Part model, mm, in its own coordinate system. Face numbers are marked on the shaded views. Give positions to 0.01 mm unless a question says otherwise; leave off trailing zeros. Order: outer loops, then holes, each group sorted by start corner. A loop starts at its lowest first (then second) coordinate and runs counter-clockwise, first axis right, second up. Notation, with made-up numbers: (-39.5, -39.75) -> (1.5, -39.75) arc R21 cw to (1.5, -32.75) -> close; hole circle Ø1 at (7, 87.5). An arc over 180 degrees is marked (long way). Write item = value, one per line. Start each with the question number.
(1) Two-plate mould, pull along Z, no slides. Class the marked faces 1, 2 and 3: pulls with the +Z half, pulls with the -Z half, needs draft (parallel to the pull), parting line crosses it, or undercut.
(2) Saw through at B-B, the plane x = -10. List the corners of the cut face in (y, z), then the cut area to 3 significant figures.
(3) Saw through at A-A, the plane x = 10. List the corners of the cut face in (y, z), then the cut area to 3 significant figures.
(4) Flat gauge pins, fed straight in: pin 1 (8 mm diameter, centred on x = 10, z = 0, fed in from +Y); pin 2 (3 mm diameter, centred on x = 10.5, z = -14.5, fed in from +Y); pin 3 (12.5 mm diameter, centred on x = 10, z = 0, fed in from -Y). Where does each tip first touch, or does it go through?
(5) Probe line 1 along X through (y, z) = (49, 0); line 2 along X through (y, z) = (47.25, 0); line 3 along Y through (x, z) = (-9.5, -6). List the from-to ranges inside material, lowest first. Write a range as from..to.
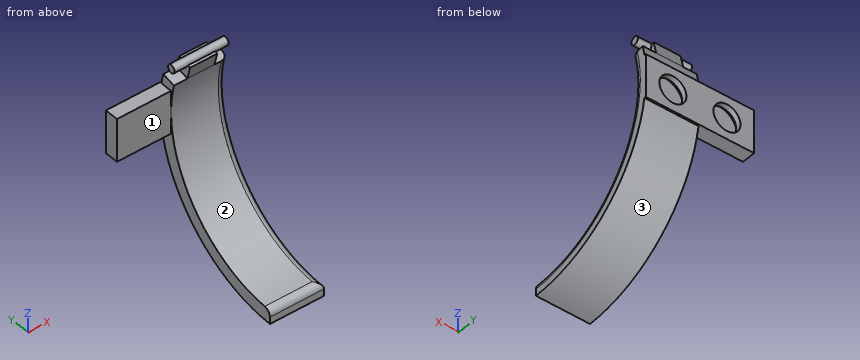
from build123d import *

# Parameters (mm, degrees)
BOSS_EXTRUDE1_DEPTH      = 20
BOSS_EXTRUDE2_DEPTH      = 20
BOSS_EXTRUDE2_DEPTH_BACK = 20
SKETCH4_R                = 5
CUT_EXTRUDE1_DEPTH       = 2
SKETCH5_R                = 7
CUT_EXTRUDE2_DEPTH       = 2
SKETCH16_W               = 20
SKETCH16_H               = 5
SKETCH17_W               = 5
SKETCH17_H               = 5
BOSS_EXTRUDE10_DEPTH     = 5
SKETCH18_R               = 1.5
BOSS_EXTRUDE11_DEPTH     = 10
SKETCH19_R               = 5
CUT_EXTRUDE3_DEPTH       = 2
SKETCH20_R               = 7
CUT_EXTRUDE4_DEPTH       = 2
FILLET2_R                = 2.5


with BuildPart() as part:
    # Sketch2 → Boss-Extrude1 (new body)
    with BuildSketch(Plane(origin=(0, 0, 0), x_dir=(0, 0, -1), z_dir=(1, 0, 0))):
        with BuildLine():
            Line((-50, 0), (-45, 0))
            ThreePointArc((-45, 0), (0, 45), (45, 0))
            Line((45, 0), (50, 0))
            ThreePointArc((50, 0), (0, 50), (-50, 0))
        make_face()
    extrude(amount=BOSS_EXTRUDE1_DEPTH)

    # Sketch3 → Boss-Extrude2 (add, two sides: drawn at the far end of the back side and taken through both)
    with BuildSketch(Plane(origin=(0, 0, 0), x_dir=(0, 0, -1), z_dir=(1, 0, 0)).offset(-BOSS_EXTRUDE2_DEPTH_BACK)):
        Polygon((0, 45), (8, 45), (8, 50), (-8, 50), (-8, 45), align=None)
    extrude(amount=BOSS_EXTRUDE2_DEPTH + BOSS_EXTRUDE2_DEPTH_BACK)

    # Sketch4 → Cut-Extrude1 (cut)
    with BuildSketch(Plane(origin=(0, 50, 0), x_dir=(1, 0, 0), z_dir=(0, 1, 0))):
        with Locations(Location((10, 0, 0), (0, 0, 270))):
            Circle(SKETCH4_R)
    extrude(amount=-CUT_EXTRUDE1_DEPTH, mode=Mode.SUBTRACT)

    # Sketch5 → Cut-Extrude2 (cut)
    with BuildSketch(Plane(origin=(0, 48, 0), x_dir=(1, 0, 0), z_dir=(0, 1, 0))):
        with Locations(Location((10, 0, 0), (0, 0, 270))):
            Circle(SKETCH5_R)
    extrude(amount=-CUT_EXTRUDE2_DEPTH, mode=Mode.SUBTRACT)

    # Cut-Sweep1: sweep along a path in Sketch15
    with BuildLine(Plane.ZY) as cut_sweep1_path:
        ThreePointArc((50, 0), (39.37003937, 30.822070015), (12, 48.538644398))
    # Sketch16 → Cut-Sweep1 (sweep, cut)
    with BuildSketch(Plane.XZ):
        with Locations((10, 47.5)):
            Rectangle(SKETCH16_W, SKETCH16_H)
    sweep(path=cut_sweep1_path.line, mode=Mode.SUBTRACT)

    # Sketch17 → Boss-Extrude10 (add)
    with BuildSketch(Plane(origin=(0, 0, 0), x_dir=(1, 0, 0), z_dir=(0, -0.24000000000000005, 0.9707728879609278))):
        with Locations((7.5, 47.5)):
            Rectangle(SKETCH17_W, SKETCH17_H)
    boss_extrude10 = extrude(amount=BOSS_EXTRUDE10_DEPTH)

    # Sketch18 → Boss-Extrude11 (add)
    with BuildSketch(Plane(origin=(10, 0, 0), x_dir=(0, 0, -1), z_dir=(1, 0, 0))):
        with Locations((-16.25386444, 44.911712178)):
            Circle(SKETCH18_R)
    boss_extrude11 = extrude(amount=-BOSS_EXTRUDE11_DEPTH)

    # Mirror1: Boss-Extrude10, Boss-Extrude11 across plane
    add(boss_extrude10.mirror(Plane(origin=(10, 42.484779958, 15.65386444), x_dir=(0, 0, 1), z_dir=(-1, 0, 0))))
    add(boss_extrude11.mirror(Plane(origin=(10, 42.484779958, 15.65386444), x_dir=(0, 0, 1), z_dir=(-1, 0, 0))))

    # Sketch19 → Cut-Extrude3 (cut)
    with BuildSketch(Plane(origin=(0, 50, 0), x_dir=(1, 0, 0), z_dir=(0, 1, 0))):
        with Locations(Location((-10, 0, 0), (0, 0, 270))):
            Circle(SKETCH19_R)
    extrude(amount=-CUT_EXTRUDE3_DEPTH, mode=Mode.SUBTRACT)

    # Sketch20 → Cut-Extrude4 (cut)
    with BuildSketch(Plane(origin=(0, 48, 0), x_dir=(1, 0, 0), z_dir=(0, 1, 0))):
        with Locations(Location((-10, 0, 0), (0, 0, 270))):
            Circle(SKETCH20_R)
    extrude(amount=-CUT_EXTRUDE4_DEPTH, mode=Mode.SUBTRACT)

    # Fillet2
    fillet2_edges = [part.edges().sort_by_distance(p)[0] for p in [
        (20, 35.433035433, -27.739863013),
        (10, 0, -45),
    ]]
    fillet(fillet2_edges, radius=FILLET2_R)


solid = part.part
Results list:
q1.face_1 = needs draft
q1.face_2 = undercut
q1.face_3 = pulls with the -Z half
q2.outline = (45, -8) -> (50, -8) -> (50, -5) -> (48, -5) -> (48, -7) -> (46, -7) -> (46, 7) -> (48, 7) -> (48, 5) -> (50, 5) -> (50, 8) -> (45, 8) -> close
q2.area = 32.0 mm^2
q3.outline = (0, -50) arc R50 ccw to (49.36, -8) -> (50, -8) -> (50, -5) -> (48, -5) -> (48, -7) -> (46, -7) -> (46, 7) -> (48, 7) -> (48, 5) -> (50, 5) -> (50, 8) -> (49.36, 8) arc R50 ccw to (48.54, 12) -> (47.34, 16.85) -> (46.37, 16.61) arc R1.5 ccw to (43.46, 15.89) -> (42.48, 15.65) -> (43.68, 10.8) arc R45 cw to (2.37, -44.94) arc R2.5 ccw to (0, -47.43) -> close
q3.area = 413 mm^2
q4.pin_1 = 46
q4.pin_2 = 48.28
q4.pin_3 = 44.56
q5.line_1 = -20..-15, -5..5, 15..20
q5.line_2 = -20..-17, -3..3, 17..19.99
q5.line_3 = 45..46, 48..50
